Geometry check sheet. Reference: the model listing, model coordinates, mm. Coordinates: 2 decimals unless noted, no trailing zeros. Write each loop counter-clockwise with the first axis right and the second up, starting at its lowest first coordinate (ties: lowest second). Pieces come first, ordered by that corner, then holes. Notation, with made-up numbers: (-3.5, -23.75) -> (50.5, -23.75) arc R13 ccw to (50.5, -1.75) -> close; hole circle Ø10 at (82.25, 40). An arc over 180 degrees is marked (long way). Put each result on its own line as item: value. Start each with the question number.
from build123d import *

# Parameters (mm, degrees)
SKETCH1_R           = 1.25
BOSS_EXTRUDE1_DEPTH = 0.675
SKETCH2_W           = 7.5
SKETCH2_H           = 10.6
BOSS_EXTRUDE2_DEPTH = 1
CUT_EXTRUDE1_DEPTH  = 3.35


with BuildPart() as part:
    # Sketch1 → Boss-Extrude1 (new body)
    with BuildSketch(Plane.XY):
        Polygon((-66.8, 18.75), (-64.3, 18.75), (-64.3, 15.8), (-66.8, 15.8), (-66.8, 11.05), (-64.3, 11.05), (-64.3, 8.1), (-66.8, 8.1), (-66.8, 1), (-65.8, 0), (0, 0), (0, 29.95), (-66.8, 29.95), align=None)
        with Locations((-64.8, 2)):
            Circle(SKETCH1_R, mode=Mode.SUBTRACT)
    extrude(amount=BOSS_EXTRUDE1_DEPTH)

    # Sketch2 → Boss-Extrude2 (add)
    with BuildSketch(Plane.XY.offset(0.675)):
        with Locations((-53.55, 17.7)):
            Rectangle(SKETCH2_W, SKETCH2_H)
        with Locations((-38.75, 17.7)):
            Rectangle(SKETCH2_W, SKETCH2_H)
        with Locations((-23.95, 17.7)):
            Rectangle(SKETCH2_W, SKETCH2_H)
        with Locations((-9.15, 17.7)):
            Rectangle(SKETCH2_W, SKETCH2_H)
    extrude(amount=BOSS_EXTRUDE2_DEPTH)

    # Mirror1: part across plane


with BuildPart() as part_1:
    add(part.part)
    add(part.part.mirror(Plane.XY))

    # Mirror2: part across plane


with BuildPart() as part_2:
    add(part_1.part)
    add(part_1.part.mirror(Plane(origin=(0, 0, 0), x_dir=(0, 0, 1), z_dir=(1, 0, 0))))

    # Sketch3 → Cut-Extrude1 (cut, through all)
    with BuildSketch(Plane.XY.offset(0.675)):
        with BuildLine():
            Line((-12.45, 0), (-12.45, 3.3))
            ThreePointArc((-12.45, 3.3), (-11.7, 4.05), (-10.95, 3.3))
            Line((-10.95, 3.3), (-10.95, 0))
            Line((-10.95, 0), (-12.45, 0))
        make_face()
    extrude(amount=-CUT_EXTRUDE1_DEPTH, mode=Mode.SUBTRACT)


solid = part_2.part
Item 1: Mould release check, pull along X, two halves, no side actions. Record for faces 1 (the flat face through (1, 15, -0.675)), 2 (the flat face through (54, 18, -1.675)): released by +X, released by -X, zero draft, split by the parting line, or undercut.
Item 2: Section check A-A, the plane x = 8.5. Enter the section's corners in (y, z) (3 decimals), and give its area (3 significant figures).
Item 3: Scan lines: line 1 along Y through (x, z) = (-64.8, 0.45); line 2 along X through (y, z) = (3, 0.1); line 3 along Z through (x, y) = (-30, 23) (3 decimals). Record each from-to range of solid material in increasing order. Write a range as [from, to].
Item 4: Section check B-B, the plane y = 26.75. Enter the section's corners in (x, z) (3 decimals), and give its area (3 significant figures).
Item 5: Go/stop test with flat-tipped pins: P1, Ø6, axis at x = 38, y = 6, coming from the -Z side (3 decimals); P2, Ø0.8, axis at x = 54, z = -1, coming from the -Y side; P3, Ø1.1, axis at y = 9, z = 0, coming from the +X side; P4, Ø0.5, axis at y = 19, z = -1.5, coming from the +X side. Record where each tip stops, or that it passes through.
From the geometry:
1. face 1: undercut
1. face 2: zero draft
2. outline: (0, -0.675) -> (12.4, -0.675) -> (12.4, -1.675) -> (23, -1.675) -> (23, -0.675) -> (29.95, -0.675) -> (29.95, 0.675) -> (23, 0.675) -> (23, 1.675) -> (12.4, 1.675) -> (12.4, 0.675) -> (0, 0.675) -> close
2. area: 61.6 mm²
3. line 1: [0, 0.75], [3.25, 8.1], [11.05, 15.8], [18.75, 29.95]
3. line 2: [-66.8, -65.55], [-64.05, -12.45], [-10.95, 64.05], [65.55, 66.8]
3. line 3: [-0.675, 0.675]
4. outline: (-66.8, -0.675) -> (66.8, -0.675) -> (66.8, 0.675) -> (-66.8, 0.675) -> close
4. area: 180 mm²
5. P1: z = -0.675
5. P2: y = 0
5. P3: x = 64.3
5. P4: x = 57.3
